Work out the finished part from the listing and answer in its coordinate system (mm). Coordinates: 2 decimals unless noted, no trailing zeros. Write each loop counter-clockwise with the first axis right and the second up, starting at its lowest first coordinate (ties: lowest second). Pieces come first, ordered by that corner, then holes. Notation, with made-up numbers: (82, 40) - (127, 40) arc R6 ccw to (127, 50) - close; hole circle Ø5 at (67, -34.5). An arc over 180 degrees is marked (long way). Use CSV: the item, a comma, the result in double quotes. Start each with the question number.
from build123d import *

# Parameters (mm, degrees)
F1_DEPTH = 20
F2_R     = 3
F2_R_2   = 4
F3_DEPTH = 20
F4_R     = 4
F5_DEPTH = 30
F6_R     = 16
F7_DEPTH = 25


with BuildPart() as f1:
    # F0 (on Front) → F1 (new body)
    with BuildSketch(Plane.XZ):
        Polygon((0, 490), (0, 0), (320, 0), (320, 90), (100, 280), (100, 490), align=None)
    extrude(amount=F1_DEPTH)

    # F2 (on face) → F3 (cut)
    with BuildSketch(Plane.XZ.offset(20)):
        with Locations((148, 26.596917)):
            Circle(F2_R)
        with Locations((148, 74.596917)):
            Circle(F2_R)
        with Locations((173, 74.596917)):
            Circle(F2_R)
        with Locations((173, 26.596917)):
            Circle(F2_R)
        with Locations((20, 470)):
            Circle(F2_R_2)
        with Locations((20, 430)):
            Circle(F2_R_2)
        with Locations((40, 390)):
            Circle(F2_R_2)
        with Locations((80, 390)):
            Circle(F2_R_2)
        with Locations((40, 350)):
            Circle(F2_R_2)
        with Locations((80, 350)):
            Circle(F2_R_2)
    extrude(amount=-F3_DEPTH, mode=Mode.SUBTRACT)

    # F4 (on face) → F5 (cut)
    with BuildSketch(Plane(origin=(0, 0, 0), x_dir=(1, 0, 0), z_dir=(0, 0, -1))):
        with Locations((35, 10)):
            Circle(F4_R)
        with Locations((95, 10)):
            Circle(F4_R)
        with Locations((160, 10)):
            Circle(F4_R)
        with Locations((225, 10)):
            Circle(F4_R)
        with Locations((285, 10)):
            Circle(F4_R)
    extrude(amount=-F5_DEPTH, mode=Mode.SUBTRACT)

    # F6 (on face) → F7 (cut)
    with BuildSketch(Plane.XZ.offset(20)):
        with Locations((70.1391, 445)):
            Circle(F6_R)
    extrude(amount=-F7_DEPTH, mode=Mode.SUBTRACT)


solid = f1.part
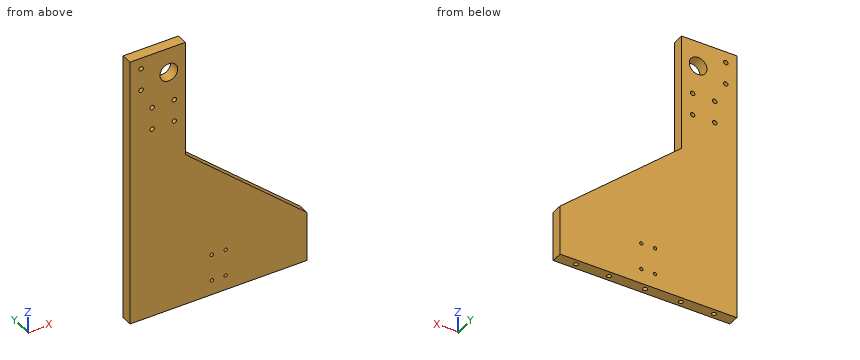
Item 1: Straight lines are drawn through the part: probe 1 along X at (y, z) = (-13.25, 350); probe 2 along Z at (x, y) = (20, -13.75); probe 3 along X at (y, z) = (-8.5, 470). For each, find the intervals that lie inside material, in ascending order. Write a range as [from, to].
Item 2: A cutting plane is placed at A-A (x = 61.5). Determine the outline of the cut face in (y, z), then the cut area to 3 significant figures.
Item 3: A cutting plane is placed at C-C (z = 261.5). Determine the outline of the cut face in (x, y), then the cut area to 3 significant figures.
Item 4: A cutting plane is placed at D-D (x = 247.5). Determine the outline of the cut face in (y, z), then the cut area to 3 significant figures.
Item 5: A cutting plane is placed at B-B (y = -10). Count the separate pieces of the cut face and the enclosed holes in it, then the cut area to 3 significant figures.
Item 6: Each of these flat-tipped pins is pushed along its axis until it touches: pin 1 (2.5 mm diameter, centred on x = 36, y = -11.5, fed in from -Z); pin 2 (6 mm diameter, centred on y = -12.5, z = 303.5, fed in from +X); pin 3 (6 mm diameter, centred on y = -4.5, z = 101.5, fed in from +X); pin 4 (5 mm diameter, centred on x = 173, z = 26.6, fed in from -Y). Where does it stop, or does it pass through?
Calculated:
1,probe 1,"x = [0, 36], [44, 76], [84, 100]"
1,probe 2,"z = [0, 426], [434, 466], [474, 490]"
1,probe 3,"x = [0, 16], [24, 100]"
2,outline,"(-20, 0) - (0, 0) - (0, 431.53) - (-20, 431.53) - close; (-20, 458.47) - (0, 458.47) - (0, 490) - (-20, 490) - close"
2,area,"9,260 mm²"
3,outline,"(0, -20) - (121.42, -20) - (121.42, 0) - (0, 0) - close"
3,area,"2,430 mm²"
4,outline,"(-20, 0) - (0, 0) - (0, 152.61) - (-20, 152.61) - close"
4,area,"3,050 mm²"
5,separate pieces,"1"
5,enclosed holes,"11"
5,area,"87,300 mm²"
6,pin 1,"stops at z = 30"
6,pin 2,"stops at x = 100"
6,pin 3,"stops at x = 310.16"
6,pin 4,"passes through"
